Input: dimensioned drawing with shaded views. Units: mm. Origin: part minimum x, y, z. A direction names the side the tool comes from. Round coordinates to 2 decimals unless told otherwise and drop trailing zeros. Loops run counter-clockwise (first coordinate to the right, second up) from the corner with the lowest first, then second, coordinate; pieces in that order, holes last. Notation, with made-up numbers: M 52,-36.75 L 56,-36.75 A17 ccw 56,-28.75 Z; hole C 88,-10.5 d10. An arc over 180 degrees is marked long. One line per item, written item: value.
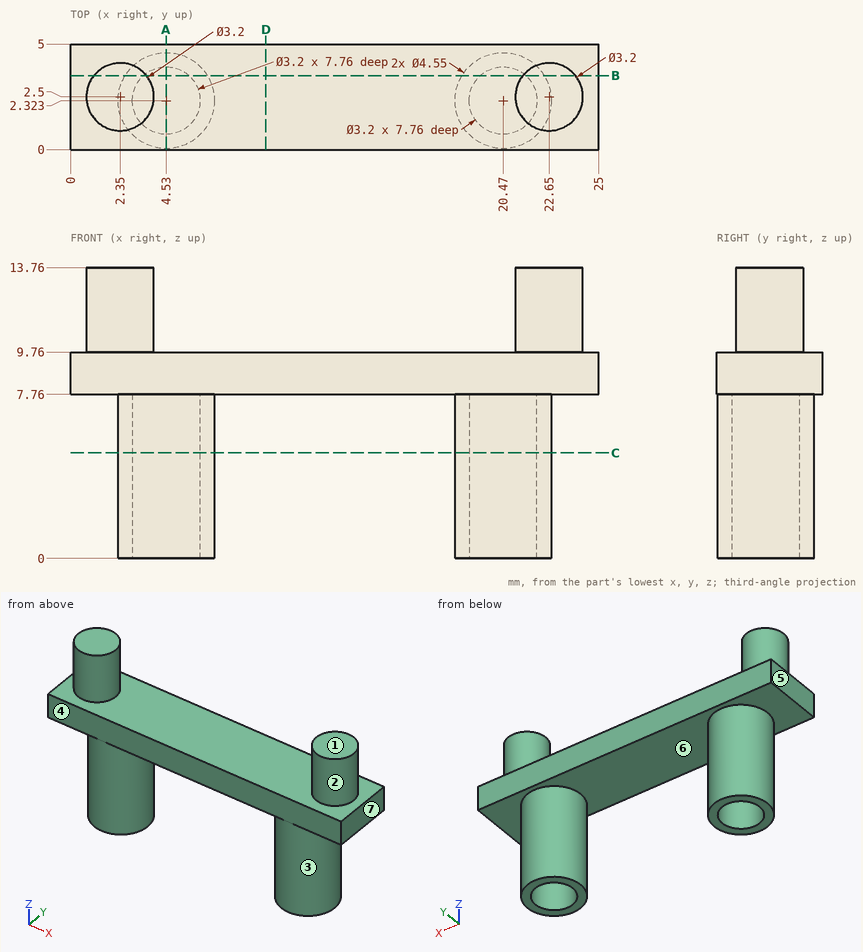
1. Pin query (flat end, axial travel): pin 1 (6 mm diameter, centred on x = 7.5, z = 4, fed in from -Y); pin 2 (1.9 mm diameter, centred on x = 4.53, y = 2.32, fed in from -Z); pin 3 (1.5 mm diameter, centred on y = 2, z = 5.5, fed in from +X) (3 decimals); pin 4 (4 mm diameter, centred on x = 14.5, z = 5, fed in from +Y). Return the tip coordinate at first contact, or that it passes through.
Report:
pin 1: stops at y = 0.05
pin 2: stops at z = 7.76
pin 3: stops at x = 22.745
pin 4: passes through
2. Pull-direction query (X, two-part tool) for the marked faces 4, 5, 6 and 7; classes: released by +X, released by -X, zero draft, split by the parting line, or undercut.
Report:
face 4: zero draft
face 5: released by -X
face 6: undercut
face 7: released by +X
3. Ray query, line 1 (X direction, y = 2.3, z = 3.5); line 2 (Y direction, x = 20.47, z = 6); line 3 (X direction, y = 2.85, z = 7). Return the intervals inside material, ascending. Write a range as [from, to].
Report:
line 1: x = [2.26, 2.93], [6.13, 6.8], [18.2, 18.87], [22.07, 22.74]
line 2: y = [0.05, 0.72], [3.92, 4.6]
line 3: x = [2.32, 3.02], [6.04, 6.74], [18.26, 18.96], [21.98, 22.68]
4. Section query A-A (x = 4.53). Return the cut outline in (y, z), and give its area (3 significant figures).
Report:
outline: M 0,7.76 L 0.05,7.76 L 0.05,0 L 0.72,0 L 0.72,7.76 L 3.92,7.76 L 3.92,0 L 4.6,0 L 4.6,7.76 L 5,7.76 L 5,9.76 L 0,9.76 Z
area: 20.5 mm2
5. Section query D-D (x = 9.25). Return the cut outline in (y, z).
Report:
outline: M 0,7.76 L 5,7.76 L 5,9.76 L 0,9.76 Z
6. Reachability of the marked faces 1, 2 and 3 from +Z, -Z, +X, -X, +Y, -Y: full face, straight path, thin tool, end or side. Return the list, or none.
Report:
face 1: +Z, +X, -X, +Y, -Y
face 2: +Z
face 3: -Z
7. Section query C-C (z = 5). Return the cut outline in (x, y) (3 decimals), and give its area (3 significant figures).
Report:
outline: C 4.53,2.323 d4.55; C 20.47,2.323 d4.55; hole C 4.53,2.323 d3.2; hole C 20.47,2.323 d3.2
area: 16.4 mm2
8. Section query B-B (y = 3.5). Return the cut outline in (x, z).
Report:
outline: M 0,7.76 L 2.58,7.76 L 2.58,0 L 3.45,0 L 3.45,7.76 L 5.61,7.76 L 5.61,0 L 6.48,0 L 6.48,7.76 L 18.52,7.76 L 18.52,0 L 19.39,0 L 19.39,7.76 L 21.55,7.76 L 21.55,0 L 22.42,0 L 22.42,7.76 L 25,7.76 L 25,9.76 L 23.9,9.76 L 23.9,13.76 L 21.4,13.76 L 21.4,9.76 L 3.6,9.76 L 3.6,13.76 L 1.1,13.76 L 1.1,9.76 L 0,9.76 Z
